```python
from build123d import *

# Parameters (mm, degrees)
BOSS_EXTRUDE1_DEPTH      = 3
BOSS_EXTRUDE1_DEPTH_BACK = 3
BOSS_EXTRUDE2_DEPTH      = 3
BOSS_EXTRUDE3_DEPTH      = 3
SKETCH4_W                = 20
SKETCH4_H                = 20
BOSS_EXTRUDE4_DEPTH      = 2


with BuildPart() as part:
    # Sketch1 → Boss-Extrude1 (new, two sides: drawn at the far end of the back side and taken through both)
    with BuildSketch(Plane(origin=(0, 0, 0), x_dir=(0, 0, -1), z_dir=(1, 0, 0)).offset(-BOSS_EXTRUDE1_DEPTH_BACK)):
        with BuildLine():
            Line((-5.5, 0), (-3.5, 0))
            ThreePointArc((-3.5, 0), (0, 3.5), (3.5, 0))
            ThreePointArc((3.5, 0), (3.446827136, -0.607768622), (3.288924173, -1.197070502))
            Line((3.288924173, -1.197070502), (5.168309414, -1.881110788))
            ThreePointArc((5.168309414, -1.881110788), (5.416442642, -0.955064977), (5.5, 0))
            ThreePointArc((5.5, 0), (0, 5.5), (-5.5, 0))
        make_face()
        with BuildLine():
            Line((5.168309414, -1.881110788), (3.288924173, -1.197070502))
            ThreePointArc((3.288924173, -1.197070502), (3.88659665, -2.478783266), (5.168309414, -1.881110788))
        make_face()
        with BuildLine():
            ThreePointArc((-3.288924173, -1.197070502), (-3.446827136, -0.607768622), (-3.5, 0))
            Line((-3.5, 0), (-5.5, 0))
            ThreePointArc((-5.5, 0), (-5.416442642, -0.955064977), (-5.168309414, -1.881110788))
            Line((-5.168309414, -1.881110788), (-4.228616794, -1.539090645))
            Line((-4.228616794, -1.539090645), (-3.288924173, -1.197070502))
        make_face()
        with BuildLine():
            ThreePointArc((-5.168309414, -1.881110788), (-3.88659665, -2.478783266), (-3.288924173, -1.197070502))
            Line((-3.288924173, -1.197070502), (-4.228616794, -1.539090645))
            Line((-4.228616794, -1.539090645), (-5.168309414, -1.881110788))
        make_face()
    extrude(amount=BOSS_EXTRUDE1_DEPTH + BOSS_EXTRUDE1_DEPTH_BACK)

    # Sketch2 → Boss-Extrude2 (add)
    with BuildSketch(Plane(origin=(0, 0, 0), x_dir=(0, 0, -1), z_dir=(1, 0, 0))):
        Polygon((-1, 3.5), (0, 3.5), (1, 3.5), (1, 46.5), (-1, 46.5), align=None)
    extrude(amount=BOSS_EXTRUDE2_DEPTH)

    # Sketch3 → Boss-Extrude3 (add)
    with BuildSketch(Plane(origin=(0, 0, 0), x_dir=(0, 0, -1), z_dir=(1, 0, 0))):
        Polygon((1, 46.5), (0, 46.5), (-1, 46.5), (-1, 3.5), (1, 3.5), align=None)
    extrude(amount=-BOSS_EXTRUDE3_DEPTH)

    # Sketch4 → Boss-Extrude4 (add)
    with BuildSketch(Plane(origin=(0, 46.5, 0), x_dir=(1, 0, 0), z_dir=(0, 1, 0))):
        Rectangle(SKETCH4_W, SKETCH4_H)
    extrude(amount=BOSS_EXTRUDE4_DEPTH)


solid = part.part
```
Verification items for the finished model (mm, model axes). A direction names the side the tool comes from. Round coordinates to 2 decimals unless told otherwise and drop trailing zeros. Order: outer loops, then holes, each group sorted by start corner. A loop starts at its lowest first (then second) coordinate and runs counter-clockwise, first axis right, second up. Notation, with made-up numbers: (-13.75, 41) - (-8.75, 41) arc R14 cw to (-8.75, 50) - close; hole circle Ø11 at (54.5, 26). An arc over 180 degrees is marked (long way). Use CSV: the item, a comma, the result in double quotes.
(1) Gauge pin test, flat ends, axial feed: pin 1 Ø3.5 at (y, z) = (13, -0.5) entering from -X; pin 2 Ø6 at (y, z) = (3, 6) entering from +X; pin 3 Ø4 at (x, y) = (-4, 5) entering from +Z; pin 4 Ø10 at (y, z) = (22.5, -7.5) entering from +X. Record the tip position at first contact, or that the pin passes through.
Entries:
pin 1,"x = -3"
pin 2,"x = 3"
pin 3,"z = 4.42"
pin 4,"through"
(2) Thickness scan on probe 1 along Y at (x, z) = (-3, -7); probe 2 along Z at (x, y) = (2.75, 44.5); probe 3 along Y at (x, z) = (1.5, 4). Record the ranges inside material, lowest first. Write a range as from..to.
Entries:
probe 1,"46.5..48.5"
probe 2,"-1..1"
probe 3,"-2.51..3.77, 46.5..48.5"
(3) Mould release check, pull along Y, two halves, no side actions. Record for faces 5 (the face through (0, 47, -10)), 6 (the face through (0, 48.5, 0)), 7 (the face through (0, 26, -1)): released by +Y, released by -Y, zero draft, split by the parting line, or undercut.
Entries:
face 5,"zero draft"
face 6,"released by +Y"
face 7,"undercut"
(4) Section check B-B on z = 0. Record the boundary of the cut face in (x, y), and give its area (3 significant figures).
Entries:
outline,"(-10, 46.5) - (-3, 46.5) - (-3, 3.5) - (3, 3.5) - (3, 46.5) - (10, 46.5) - (10, 48.5) - (-10, 48.5) - close"
area,"298 mm^2"
(5) Access from +Z, -Z, +X, -X, +Y, -Y to the whole of each face (thin tool, end or side, straight path). Record for faces 1 (the face through (-3, 18, 0)), 2 (the face through (3, 18, 0)), 3 (the face through (-10, 47, 0)), 4 (the face through (0, 26, 1)).
Entries:
face 1,"+Z, -Z, -X, -Y"
face 2,"+Z, -Z, +X, -Y"
face 3,"+Z, -Z, -X, +Y, -Y"
face 4,"+Z, +X, -X"
(6) Section check A-A on x = -1.5. Record the boundary of the cut face in (y, z).
Entries:
outline,"(-1.88, -5.17) arc R5.5 ccw to (5.41, -1) - (46.5, -1) - (46.5, -10) - (48.5, -10) - (48.5, 10) - (46.5, 10) - (46.5, 1) - (5.41, 1) arc R5.5 ccw to (-1.88, 5.17) arc R1 ccw to (-1.2, 3.29) arc R3.5 cw (long way) to (-1.2, -3.29) arc R1 ccw to start"
(7) Section check C-C on y = 20. Record the boundary of the cut face in (x, z), and give its area (3 significant figures).
Entries:
outline,"(-3, -1) - (3, -1) - (3, 1) - (-3, 1) - close"
area,"12.0 mm^2"
(8) Section check D-D on z = 7.5. Record the boundary of the cut face in (x, y), and give its area (3 significant figures).
Entries:
outline,"(-10, 46.5) - (10, 46.5) - (10, 48.5) - (-10, 48.5) - close"
area,"40.0 mm^2"
